Source: CAD feature listing. Evaluate the final solid. Frame: model axes, mm. Face numbers are marked on the shaded views. A direction names the side the tool comes from. Coordinates: 2 decimals unless noted, no trailing zeros. Order: outer loops, then holes, each group sorted by start corner. A loop starts at its lowest first (then second) coordinate and runs counter-clockwise, first axis right, second up.
```python
from build123d import *

# Parameters (mm, degrees)
BOSS_EXTRUDE1_DEPTH     = 10
FILLET1_R               = 2
BOSS_EXTRUDE2_START     = 10
SKETCH1_3_R             = 22.5
SKETCH1_3_R_2           = 20
SKETCH1_3_R_3           = 2.5
BOSS_EXTRUDE2_DEPTH     = 7.5
SKETCH2_R               = 2.1
CUT_EXTRUDE2_DEPTH      = 17.5
CIRPATTERN1_START       = 10
CIRPATTERN1_OUTLINE_R   = 2.1
CIRPATTERN1_DEPTH       = 7.5
CIRPATTERN1_2_OUTLINE_R = 2.1
CIRPATTERN1_2_DEPTH     = 10


# Read off the part's stored shape, not the designer's step: CirPattern1
with BuildPart() as part:
    # Sketch1 → Boss-Extrude1 (new body)
    with BuildSketch(Plane.XY):
        with BuildLine():
            ThreePointArc((6.867732558, 8.910485369), (9.742785793, 5.625), (11.150572969, 1.492388177))
            Line((11.150572969, 1.492388177), (19.823240833, 2.653134537))
            ThreePointArc((19.823240833, 2.653134537), (17.320508076, 10), (12.209302326, 15.840862878))
            Line((12.209302326, 15.840862878), (6.867732558, 8.910485369))
        make_face()
    extrude(amount=BOSS_EXTRUDE1_DEPTH)

    # Fillet1
    fillet1_edges = [part.edges().sort_by_distance(p)[0] for p in [
        (11.150572969, 1.492388177, 5),
        (6.867732558, 8.910485369, 5),
        (12.209302326, 15.840862878, 5),
        (19.823240833, 2.653134537, 5),
    ]]
    fillet(fillet1_edges, radius=FILLET1_R)

    # Sketch1<3> → Boss-Extrude2 (add)
    # profile 1 of 3: a face of its own
    with BuildSketch(Plane.XY.offset(BOSS_EXTRUDE2_START)):
        Circle(SKETCH1_3_R)
        Circle(SKETCH1_3_R_2, mode=Mode.SUBTRACT)
    # profile 2 of 3: a face of its own
    with BuildSketch(Plane.XY.offset(BOSS_EXTRUDE2_START)):
        with BuildLine():
            Line((19.823240833, 2.653134537), (11.150572969, 1.492388177))
            ThreePointArc((11.150572969, 1.492388177), (11.225115721, 0.747848281), (11.25, 0))
            ThreePointArc((11.25, 0), (-10.095159515, -4.964902251), (6.867732558, 8.910485369))
            Line((6.867732558, 8.910485369), (12.209302326, 15.840862878))
            ThreePointArc((12.209302326, 15.840862878), (-17.946950249, -8.82649289), (20, 0))
            ThreePointArc((20, 0), (19.955761282, 1.329508055), (19.823240833, 2.653134537))
        make_face()
        with Locations((-14.895636945, -8.6)):
            Circle(SKETCH1_3_R_3, mode=Mode.SUBTRACT)
        with Locations((14.895636945, -8.6)):
            Circle(SKETCH1_3_R_3, mode=Mode.SUBTRACT)
        with Locations((0, 17.2)):
            Circle(SKETCH1_3_R_3, mode=Mode.SUBTRACT)
    # profile 3 of 3: a face of its own
    with BuildSketch(Plane.XY.offset(BOSS_EXTRUDE2_START)):
        with BuildLine():
            ThreePointArc((6.867732558, 8.910485369), (9.742785793, 5.625), (11.150572969, 1.492388177))
            Line((11.150572969, 1.492388177), (19.823240833, 2.653134537))
            ThreePointArc((19.823240833, 2.653134537), (17.320508076, 10), (12.209302326, 15.840862878))
            Line((12.209302326, 15.840862878), (6.867732558, 8.910485369))
        make_face()
    extrude(amount=BOSS_EXTRUDE2_DEPTH)

    # Sketch2 → Cut-Extrude2 (cut)
    with BuildSketch(Plane(origin=(0, 0, 0), x_dir=(-1, 0, 0), z_dir=(0, 0, -1))):
        with Locations((-13.531646934, 7.8125)):
            Circle(SKETCH2_R)
    extrude(amount=-CUT_EXTRUDE2_DEPTH, mode=Mode.SUBTRACT)

    # CirPattern1 outline → CirPattern1 (cut)
    with BuildSketch(Plane.XY.offset(CIRPATTERN1_START)):
        with Locations((0, -15.625)):
            Circle(CIRPATTERN1_OUTLINE_R)
        with Locations((-13.531646934, 7.8125)):
            Circle(CIRPATTERN1_OUTLINE_R)
    extrude(amount=CIRPATTERN1_DEPTH, mode=Mode.SUBTRACT)

    # CirPattern1 2 outline → CirPattern1 2 (add)
    # profile 1 of 2: a face of its own
    with BuildSketch(Plane.XY):
        with BuildLine():
            ThreePointArc((-13.893798079, 14.386186949), (-17.320508076, 10), (-19.405702401, 4.839288617))
            ThreePointArc((-19.405702401, 4.839288617), (-19.119544932, 3.231563339), (-17.730445615, 2.373035672))
            Line((-17.730445615, 2.373035672), (-12.982425667, 1.737562602))
            ThreePointArc((-12.982425667, 1.737562602), (-11.626778767, 2.043231391), (-10.797548106, 3.158394355))
            ThreePointArc((-10.797548106, 3.158394355), (-9.742785793, 5.625), (-8.1340238, 7.771753781))
            ThreePointArc((-8.1340238, 7.771753781), (-7.582879674, 9.047470081), (-7.995986187, 10.37432913))
            Line((-7.995986187, 10.37432913), (-10.920331983, 14.168498487))
            ThreePointArc((-10.920331983, 14.168498487), (-12.358388411, 14.94222995), (-13.893798079, 14.386186949))
        make_face()
        with Locations((-13.531646934, 7.8125)):
            Circle(CIRPATTERN1_2_OUTLINE_R, mode=Mode.SUBTRACT)
    # profile 2 of 2: a face of its own
    with BuildSketch(Plane.XY):
        with BuildLine():
            ThreePointArc((2.663524306, -10.930148136), (0, -11.25), (-2.663524306, -10.930148136))
            ThreePointArc((-2.663524306, -10.930148136), (-4.043899093, -11.090701472), (-4.98643948, -12.111891731))
            Line((-4.98643948, -12.111891731), (-6.810113632, -16.541534159))
            ThreePointArc((-6.810113632, -16.541534159), (-6.761156521, -18.173793289), (-5.511904322, -19.225475566))
            ThreePointArc((-5.511904322, -19.225475566), (0, -20), (5.511904322, -19.225475566))
            ThreePointArc((5.511904322, -19.225475566), (6.761156521, -18.173793289), (6.810113632, -16.541534159))
            Line((6.810113632, -16.541534159), (4.98643948, -12.111891731))
            ThreePointArc((4.98643948, -12.111891731), (4.043899093, -11.090701472), (2.663524306, -10.930148136))
        make_face()
        with Locations((0, -15.625)):
            Circle(CIRPATTERN1_2_OUTLINE_R, mode=Mode.SUBTRACT)
    extrude(amount=CIRPATTERN1_2_DEPTH)


solid = part.part
```
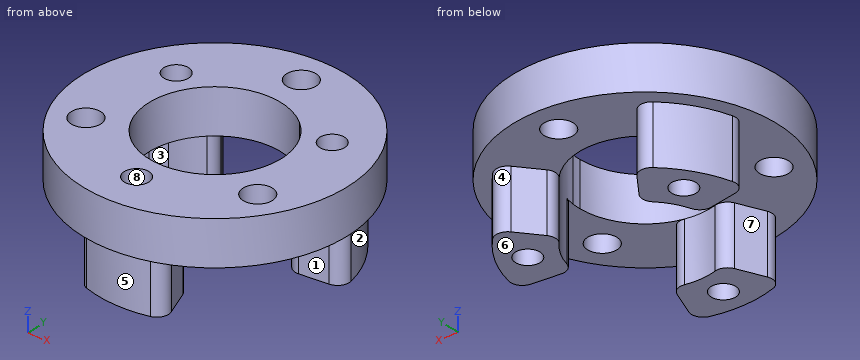
1. Section query B-B on z = 6.25. Count the separate pieces of the cut face and the enclosed holes in it, plus the area to 3 significant figures.
Findings:
separate pieces: 3
enclosed holes: 3
area: 269 mm2
2. Draft query along Y for the marked faces 5, 6, 7 and 8. Return one class per face: released by +Y, released by -Y, zero draft, split by the parting line, or undercut.
Findings:
face 5: released by -Y
face 6: zero draft
face 7: released by +Y
face 8: undercut
3. Ray query, line 1 (Y direction, x = 0, z = 12.25) (3 decimals); line 2 (Y direction, x = 0, z = 6.25) (3 decimals); line 3 (X direction, y = -9, z = 15.75). Return the intervals inside material, ascending.
Findings:
line 1: y = -22.5 to -17.725, -13.525 to -11.25, 11.25 to 14.7, 19.7 to 22.5
line 2: y = -20 to -17.725, -13.525 to -11.25
line 3: x = -20.62 to -17.36, -12.43 to -6.75, 6.75 to 12.43, 17.36 to 20.62
4. Section query C-C on y = 7. Return loops of the section in (x, z) (3 decimals).
Findings:
outline: (-21.383, 10) - (-18.735, 10) - (-18.735, 0) - (-15.468, 0) - (-15.468, 17.5) - (-21.383, 17.5) - close; (-11.595, 0) - (-8.807, 0) - (-8.807, 17.5) - (-11.595, 17.5) - close; (8.807, 0) - (11.595, 0) - (11.595, 17.5) - (8.807, 17.5) - close; (15.468, 0) - (18.735, 0) - (18.735, 10) - (21.383, 10) - (21.383, 17.5) - (15.468, 17.5) - close
5. Access query for the marked faces 1, 2, 3 and 4. Directions: +Z, -Z, +X, -X, +Y, -Y. A direction counts if a zero-diameter tool reaches every point of the face in a straight line with its end or side. Return the directions, or none.
Findings:
face 1: -Z, +X, -Y
face 2: -Z, +X, +Y
face 3: -Z, -Y
face 4: -Z, +Y
6. Pin query (flat end, axial travel): P1, Ø1, axis at x = 13.5, z = 3.5, coming from the -Y side; P2, Ø2, axis at x = 7, y = -7, coming from the +Z side; P3, Ø2, axis at y = 7, z = 2, coming from the +X side; P4, Ø1, axis at y = 15, z = 14, coming from the +X side. Return the tip coordinate at first contact, or that it passes through.
Findings:
P1: stops at y = 1.74
P2: passes through
P3: stops at x = 19.08
P4: stops at x = 17.2
7. Section query A-A on x = 0. Return loops of the section in (y, z) (3 decimals), plus the area to 3 significant figures.
Findings:
outline: (-22.5, 10) - (-20, 10) - (-20, 0) - (-17.725, 0) - (-17.725, 17.5) - (-22.5, 17.5) - close; (-13.525, 0) - (-11.25, 0) - (-11.25, 17.5) - (-13.525, 17.5) - close; (11.25, 10) - (14.7, 10) - (14.7, 17.5) - (11.25, 17.5) - close; (19.7, 10) - (22.5, 10) - (22.5, 17.5) - (19.7, 17.5) - close
area: 145 mm2
8. Section query D-D on y = 17.2. Return loops of the section in (x, z), plus the area to 3 significant figures.
Findings:
outline: (-14.51, 10) - (-2.5, 10) - (-2.5, 17.5) - (-14.51, 17.5) - close; (2.5, 10) - (14.51, 10) - (14.51, 17.5) - (2.5, 17.5) - close
area: 180 mm2
